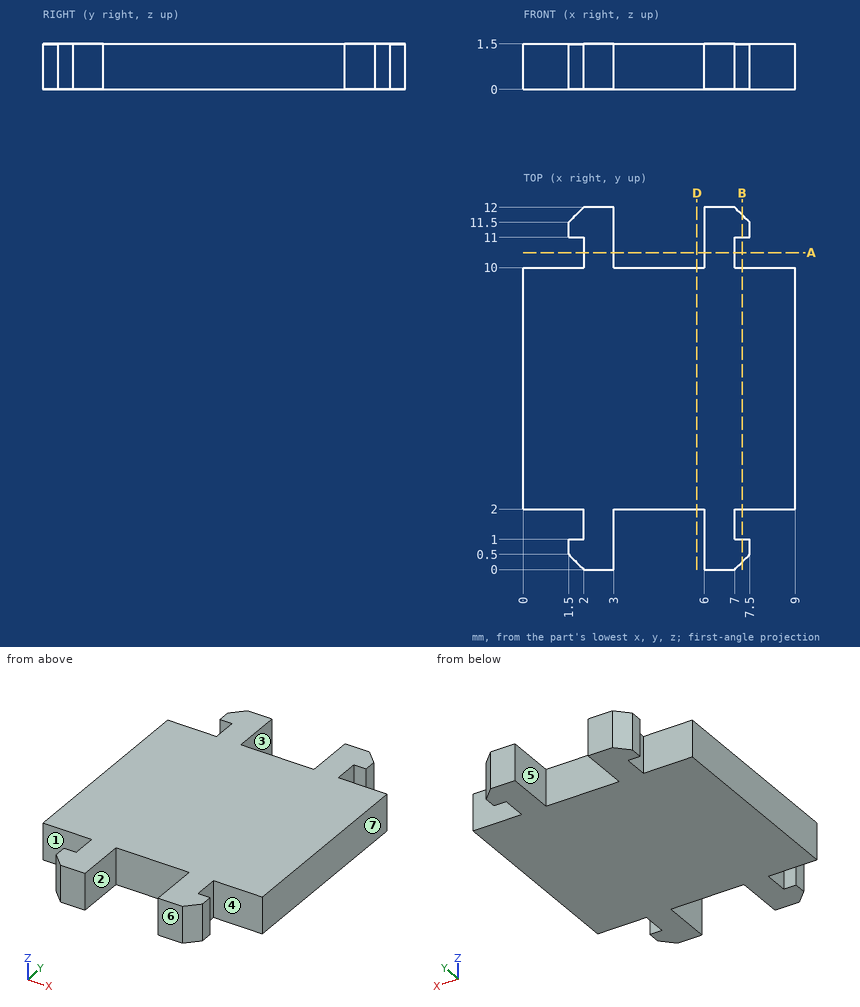
Geometry check sheet. Reference: drawing and pictorial views, mm from the part's lowest x, y, z. A direction names the side the tool comes from. Coordinates: 2 decimals unless noted, no trailing zeros. Loops run counter-clockwise (first coordinate to the right, second up) from the corner with the lowest first, then second, coordinate; pieces in that order, holes last. Notation, with made-up numbers: M 21,-21.5 L 52,-21.5 A21 cw 52,-12.5 Z; hole C 15.25,38 d9. An arc over 180 degrees is marked long. One line per item, written item: value.
1. Gauge pin test, flat ends, axial feed: P1, Ø0.8, axis at x = 8.5, z = 0.5, coming from the -Y side; P2, Ø0.5, axis at y = 10.5, z = 0.5, coming from the +X side; P3, Ø0.6, axis at y = 1, z = 0.5, coming from the -X side. Record the tip position at first contact, or that the pin passes through.
Answers follow:
P1: y = 2
P2: x = 7
P3: x = 1.5
2. Material ranges on line 1 along Y through (x, z) = (1.75, 1.05); line 2 along Y through (x, z) = (5.75, 1.05); line 3 along X through (y, z) = (10.25, 1.45), recorded low to high. Write a range as from..to.
Answers follow:
line 1: 0.25..1, 2..10, 11..11.75
line 2: 2..10
line 3: 2..3, 6..7
3. Section check B-B on x = 7.25. Record the cut outline in (y, z), plus the area to 4 significant figures.
Answers follow:
outline: M 0.25,0 L 1,0 L 1,1.5 L 0.25,1.5 Z; M 2,0 L 10,0 L 10,1.5 L 2,1.5 Z; M 11,0 L 11.75,0 L 11.75,1.5 L 11,1.5 Z
area: 14.25 mm^2
4. Section check D-D on x = 5.75. Record the cut outline in (y, z).
Answers follow:
outline: M 2,0 L 10,0 L 10,1.5 L 2,1.5 Z
5. Section check A-A on y = 10.5. Record the cut outline in (x, z), plus the area to 3 significant figures.
Answers follow:
outline: M 2,0 L 3,0 L 3,1.5 L 2,1.5 Z; M 6,0 L 7,0 L 7,1.5 L 6,1.5 Z
area: 3.00 mm^2
6. Set-up check for the marked faces 1, 2, 3 and 4: record each of +Z, -Z, +X, -X, +Y, -Y from which the full face is reachable in a straight line by a thin tool's end or side.
Answers follow:
face 1: +Z, -Z, -X
face 2: +Z, -Z, -Y
face 3: +Z, -Z, +Y
face 4: +Z, -Z, +X
7. Mould release check, pull along X, two halves, no side actions. Record for the marked faces 5, 6 and 7: pulls with the +X half, pulls with the -X half, needs draft (parallel to the pull), parting line crosses it, or undercut.
Answers follow:
face 5: undercut
face 6: needs draft
face 7: pulls with the +X half
